Read the model definition and answer for the solid it produces. Units are mm, in the model's axes. A direction names the side the tool comes from. Give positions to 0.01 mm unless a question says otherwise; leave off trailing zeros. Order: outer loops, then holes, each group sorted by start corner. A loop starts at its lowest first (then second) coordinate and runs counter-clockwise, first axis right, second up.
Item 1: Given pin 1 Ø2 at (x, y) = (3.09, 61.91) entering from -Z; pin 2 Ø4.5 at (x, y) = (97, 35.5) entering from +Z, each flat-ended and moving along its own axis, determine where each tip first touches the part or whether it passes through.
Item 2: A cutting plane is placed at C-C (x = 45). State how many separate pieces and enclosed holes the cut face has, plus the area to 3 significant figures.
Item 3: Find the intervals of material crossed by line 1 along X through (y, z) = (35.5, 9); line 2 along Y through (x, z) = (15.5, 9.8); line 3 along X through (y, z) = (2.04, 9.55), in increasing order.
Item 4: A cutting plane is placed at A-A (x = 16). Write down the section's boundary in (y, z).
Item 5: A cutting plane is placed at B-B (y = 35.5). Write down the section's boundary in (x, z), plus the area to 3 significant figures.
Item 6: Which of the six approach directions +Z, -Z, +X, -X, +Y, -Y give full straight-line access (tool end or side, diameter ignored) to faces 4 (the face through (63, 4.699, 10)), 5 (the face through (100.778, 24.712, 9.852)), 6 (the face through (76.33, 11.76, 11.37))?
Item 7: The mould has two halves that part along Y. Classify faces 1 (the face through (75.68, 7.08, 9.89)), 2 (the face through (88.505, 11.808, 9.852)), 3 (the face through (-1.2, 32, 10)): +Y half, -Y half, draft (parallel to the pull), parting line (faces both ways), or undercut.
from build123d import *

# Parameters (mm, degrees)
BOSS_EXTRUDE1_DEPTH                            = 3
CSK_FOR_M3_FLAT_HEAD_MACHINE_SCREW1_AT_2_COUNT = 2
CSK_FOR_M3_FLAT_HEAD_MACHINE_SCREW1_AT_2_PITCH = 60.801526997
CSK_FOR_M3_FLAT_HEAD_MACHINE_SCREW1_AT_3_COUNT = 2
CSK_FOR_M3_FLAT_HEAD_MACHINE_SCREW1_AT_3_PITCH = 92.34886737
CSK_FOR_M3_FLAT_HEAD_MACHINE_SCREW1_AT_4_COUNT = 2
CSK_FOR_M3_FLAT_HEAD_MACHINE_SCREW1_AT_4_PITCH = 97.558137473
CUT_EXTRUDE1_DEPTH                             = 121.966441627
SKETCH8_R                                      = 1
CUT_EXTRUDE2_DEPTH                             = 10
SKETCH10_R                                     = 1
CUT_EXTRUDE4_DEPTH                             = 10
SKETCH12_R                                     = 1.5
CUT_EXTRUDE5_DEPTH                             = 10
CHAMFER2_SIZE                                  = 0.5


with BuildPart() as part:
    # Sketch2 → Boss-Extrude1 (new body)
    with BuildSketch(Plane.XY.offset(8.62)):
        with BuildLine():
            Line((4.5, 66.2), (95.5, 66.2))
            ThreePointArc((95.5, 66.2), (99.530508653, 64.530508653), (101.2, 60.5))
            Line((101.2, 60.5), (101.2, 26.863961031))
            ThreePointArc((101.2, 26.863961031), (100.766113335, 24.682665466), (99.530508653, 22.833452378))
            Line((99.530508653, 22.833452378), (77.166547622, 0.469491347))
            ThreePointArc((77.166547622, 0.469491347), (75.317334534, -0.766113335), (73.136038969, -1.2))
            Line((73.136038969, -1.2), (4.5, -1.2))
            ThreePointArc((4.5, -1.2), (0.469491347, 0.469491347), (-1.2, 4.5))
            Line((-1.2, 4.5), (-1.2, 60.5))
            ThreePointArc((-1.2, 60.5), (0.469491347, 64.530508653), (4.5, 66.2))
        make_face()
    extrude(amount=BOSS_EXTRUDE1_DEPTH)

    # Sketch5 → CSK for M3 Flat Head Machine Screw1 (revolve, cut)
    with BuildSketch(Plane(origin=(3.085786438, 61.914213562, 11.62), x_dir=(0, -1, 0), z_dir=(1, 0, 0))):
        Polygon((0, 0), (0, 3), (1.7, 3), (1.7, 1.45), (3.15, 0), align=None)
    csk_for_m3_flat_head_machine_screw1 = revolve(axis=Axis((3.085786438, 61.914213562, 17.97), (0, 0, -1)), mode=Mode.SUBTRACT)

    # CSK for M3 Flat Head Machine Screw1 at 2: CSK for M3 Flat Head Machine Screw1 ×2
    with Locations(*[Vector(0.21239949389766488, -0.9771829178777205, 0) * (i * CSK_FOR_M3_FLAT_HEAD_MACHINE_SCREW1_AT_2_PITCH) for i in range(1, CSK_FOR_M3_FLAT_HEAD_MACHINE_SCREW1_AT_2_COUNT)]):
        add(csk_for_m3_flat_head_machine_screw1, mode=Mode.SUBTRACT)

    # CSK for M3 Flat Head Machine Screw1 at 3: CSK for M3 Flat Head Machine Screw1 ×2
    with Locations(*[Vector(0.7670014457738275, -0.6416453710429606, 0) * (i * CSK_FOR_M3_FLAT_HEAD_MACHINE_SCREW1_AT_3_PITCH) for i in range(1, CSK_FOR_M3_FLAT_HEAD_MACHINE_SCREW1_AT_3_COUNT)]):
        add(csk_for_m3_flat_head_machine_screw1, mode=Mode.SUBTRACT)

    # CSK for M3 Flat Head Machine Screw1 at 4: CSK for M3 Flat Head Machine Screw1 ×2
    with Locations(*[Vector(0.9626486933350611, -0.27075356548030866, 0) * (i * CSK_FOR_M3_FLAT_HEAD_MACHINE_SCREW1_AT_4_PITCH) for i in range(1, CSK_FOR_M3_FLAT_HEAD_MACHINE_SCREW1_AT_4_COUNT)]):
        add(csk_for_m3_flat_head_machine_screw1, mode=Mode.SUBTRACT)

    # Sketch6 → Cut-Extrude1 (cut, through all)
    with BuildSketch(Plane.XY.offset(11.62)):
        with BuildLine():
            Line((68.326, 1.397), (58.166, 1.397))
            ThreePointArc((58.166, 1.397), (56.515, 3.048), (58.166, 4.699))
            Line((58.166, 4.699), (68.326, 4.699))
            ThreePointArc((68.326, 4.699), (69.977, 3.048), (68.326, 1.397))
        make_face()
    extrude(amount=-CUT_EXTRUDE1_DEPTH, mode=Mode.SUBTRACT)

    # Sketch8 → Cut-Extrude2 (cut)
    with BuildSketch(Plane.XY.offset(11.62)):
        with Locations((44.958, 2.539999994)):
            Circle(SKETCH8_R)
        with Locations((44.958000001, 6.095999994)):
            Circle(SKETCH8_R)
    extrude(amount=-CUT_EXTRUDE2_DEPTH, mode=Mode.SUBTRACT)

    # Sketch10 → Cut-Extrude4 (cut)
    with BuildSketch(Plane.XY.offset(11.62)):
        with Locations((5.147878003, 21.843999999)):
            Circle(SKETCH10_R)
        with Locations((8.647878003, 21.843999999)):
            Circle(SKETCH10_R)
    extrude(amount=-CUT_EXTRUDE4_DEPTH, mode=Mode.SUBTRACT)

    # Sketch12 → Cut-Extrude5 (cut)
    with BuildSketch(Plane.XY.offset(11.62)):
        with Locations((44.958000001, 6.595999994)):
            Circle(SKETCH12_R)
        with Locations((44.958000001, 2.039999994)):
            Circle(SKETCH12_R)
        with BuildLine():
            Line((5.647878003, 23.343999999), (8.147878003, 23.343999999))
            ThreePointArc((8.147878003, 23.343999999), (9.647878003, 21.843999999), (8.147878003, 20.343999999))
            Line((8.147878003, 20.343999999), (5.647878003, 20.343999999))
            ThreePointArc((5.647878003, 20.343999999), (4.147878003, 21.843999999), (5.647878003, 23.343999999))
        make_face()
        with BuildLine():
            Line((69.33347303, 9.140911087), (72.256122761, 14.203088914))
            ThreePointArc((72.256122761, 14.203088914), (74.305160867, 14.752127019), (74.854198973, 12.703088914))
            Line((74.854198973, 12.703088914), (71.931549242, 7.640911087))
            ThreePointArc((71.931549242, 7.640911087), (69.882511136, 7.091872982), (69.33347303, 9.140911087))
        make_face()
        with BuildLine():
            Line((63.559970339, 9.140911087), (66.482620069, 14.203088914))
            ThreePointArc((66.482620069, 14.203088914), (68.531658175, 14.752127019), (69.080696281, 12.703088914))
            Line((69.080696281, 12.703088914), (66.15804655, 7.640911087))
            ThreePointArc((66.15804655, 7.640911087), (64.109008444, 7.091872982), (63.559970339, 9.140911087))
        make_face()
        with BuildLine():
            Line((75.106975722, 9.140911087), (78.029625453, 14.203088914))
            ThreePointArc((78.029625453, 14.203088914), (80.078663559, 14.752127019), (80.627701665, 12.703088914))
            Line((80.627701665, 12.703088914), (77.705051934, 7.640911087))
            ThreePointArc((77.705051934, 7.640911087), (75.656013828, 7.091872982), (75.106975722, 9.140911087))
        make_face()
    extrude(amount=-CUT_EXTRUDE5_DEPTH, mode=Mode.SUBTRACT)

    # Chamfer2
    chamfer2_edges = [part.edges().sort_by_distance(p)[0] for p in [
        (75.317334534, -0.766113335, 11.62),
        (4.147878003, 21.843999999, 11.62),
        (6.897878003, 20.343999999, 11.62),
        (9.647878003, 21.843999999, 11.62),
        (6.897878003, 23.343999999, 11.62),
        (43.458000001, 6.595999994, 11.62),
        (43.458000001, 2.039999994, 11.62),
        (88.348528137, 11.651471863, 11.62),
        (69.882511136, 7.091872982, 11.62),
        (73.392874107, 10.172000001, 11.62),
        (74.305160867, 14.752127019, 11.62),
        (70.794797896, 11.672000001, 11.62),
        (64.109008444, 7.091872982, 11.62),
        (67.619371415, 10.172000001, 11.62),
        (68.531658175, 14.752127019, 11.62),
        (65.021295204, 11.672000001, 11.62),
        (100.766113335, 24.682665466, 11.62),
        (75.656013828, 7.091872982, 11.62),
        (79.166376799, 10.172000001, 11.62),
        (80.078663559, 14.752127019, 11.62),
        (76.568300588, 11.672000001, 11.62),
        (101.2, 43.681980515, 11.62),
        (99.530508653, 64.530508653, 11.62),
        (50, 66.2, 11.62),
        (0.469491347, 64.530508653, 11.62),
        (-1.2, 32.5, 11.62),
        (0.469491347, 0.469491347, 11.62),
        (69.977, 3.048, 11.62),
        (63.246, 4.699, 11.62),
        (56.515, 3.048, 11.62),
        (63.246, 1.397, 11.62),
        (38.818019485, -1.2, 11.62),
    ]]
    chamfer(chamfer2_edges, length=CHAMFER2_SIZE)


solid = part.part
Response values:
1. pin 1: passes through
1. pin 2: stops at z = 10.72
2. separate pieces: 3
2. enclosed holes: 0
2. area: 183 mm2
3. line 1: x = -1.2 to 95.3, 98.7 to 101.2
3. line 2: y = -1.2 to 0.88, 4.12 to 66.2
3. line 3: x = -0.64 to 14.36, 17.64 to 43.46, 46.46 to 56.86, 69.63 to 72.33, 75.5 to 78.74
4. outline: (-1.2, 8.62) - (0.8, 8.62) - (0.8, 10.17) - (-0.65, 11.62) - (-0.7, 11.62) - (-1.2, 11.12) - close; (4.2, 8.62) - (66.2, 8.62) - (66.2, 11.12) - (65.7, 11.62) - (5.65, 11.62) - (4.2, 10.17) - close
5. outline: (-1.2, 8.62) - (95.3, 8.62) - (95.3, 10.17) - (93.85, 11.62) - (-0.7, 11.62) - (-1.2, 11.12) - close; (98.7, 8.62) - (101.2, 8.62) - (101.2, 11.12) - (100.7, 11.62) - (100.15, 11.62) - (98.7, 10.17) - close
5. area: 295 mm2
6. face 4: +Z, -Z
6. face 5: +Z, -Z, +X, -Y
6. face 6: +Z
7. face 1: undercut
7. face 2: -Y half
7. face 3: draft
